Source: CAD feature listing. Evaluate the final solid. Frame: model axes, mm. A direction names the side the tool comes from. Give positions to 0.01 mm unless a question says otherwise; leave off trailing zeros. Loops run counter-clockwise (first coordinate to the right, second up) from the corner with the lowest first, then second, coordinate; pieces in that order, holes last. Notation, with made-up numbers: M 15,74 L 38,74 A35 cw 38,110 Z; hole C 42,-37 d9. An arc over 180 degrees is marked long. Put each result on its own line as item: value.
from build123d import *

# Parameters (mm, degrees)
SKETCH_3_R             = 6
EXTRUDE_1_DEPTH        = 4
FILLET_1_R             = 2
HOLE_WIZARD_M4_2_D     = 3.3
HOLE_WIZARD_M4_2_DEPTH = 11.5
HOLE_WIZARD_M4_2_TIP   = 0.991420021


with BuildPart() as part:
    # 草图3 → 凸台-拉伸1 (new body)
    with BuildSketch(Plane.XY):
        with BuildLine():
            Line((-2.5, -27), (2.5, -27))
            ThreePointArc((2.5, -27), (3.914213562, -26.414213562), (4.5, -25))
            Line((4.5, -25), (4.5, -24.5))
            ThreePointArc((4.5, -24.5), (5.085786438, -23.085786438), (6.5, -22.5))
            Line((6.5, -22.5), (10, -22.5))
            ThreePointArc((10, -22.5), (11.414213562, -21.914213562), (12, -20.5))
            Line((12, -20.5), (12, 20.5))
            ThreePointArc((12, 20.5), (11.414213562, 21.914213562), (10, 22.5))
            Line((10, 22.5), (4.5, 22.5))
            Line((4.5, 22.5), (4.5, 25))
            ThreePointArc((4.5, 25), (3.914213562, 26.414213562), (2.5, 27))
            Line((2.5, 27), (-2.5, 27))
            ThreePointArc((-2.5, 27), (-3.914213562, 26.414213562), (-4.5, 25))
            Line((-4.5, 25), (-4.5, 22.5))
            Line((-4.5, 22.5), (-10, 22.5))
            ThreePointArc((-10, 22.5), (-11.414213562, 21.914213562), (-12, 20.5))
            Line((-12, 20.5), (-12, -20.5))
            ThreePointArc((-12, -20.5), (-11.414213562, -21.914213562), (-10, -22.5))
            Line((-10, -22.5), (-6.5, -22.5))
            ThreePointArc((-6.5, -22.5), (-5.085786438, -23.085786438), (-4.5, -24.5))
            Line((-4.5, -24.5), (-4.5, -25))
            ThreePointArc((-4.5, -25), (-3.914213562, -26.414213562), (-2.5, -27))
        make_face()
        Circle(SKETCH_3_R, mode=Mode.SUBTRACT)
    extrude(amount=EXTRUDE_1_DEPTH)

    # 草图6 → M2.5 螺纹孔1 (revolve, cut)
    with BuildSketch(Plane(origin=(0, 27, 2), x_dir=(0, 0, 1), z_dir=(1, 0, 0))):
        Polygon((0, 0), (0, 7.865882135), (1.025, 7.25), (1.025, 0), align=None)
    hole_wizard_m2_5_1 = revolve(axis=Axis((0, 33.35, 2), (0, -1, 0)), mode=Mode.SUBTRACT)

    # 镜向1: M2.5 螺纹孔1 across plane
    add(hole_wizard_m2_5_1.mirror(Plane.ZX), mode=Mode.SUBTRACT)

    # 圆角1
    fillet_1_edges = [part.edges().sort_by_distance(p)[0] for p in [
        (-4.5, 22.5, 2),
        (4.5, 22.5, 2),
    ]]
    fillet(fillet_1_edges, radius=FILLET_1_R)

    # M4 螺纹孔2
    with Locations(Plane(origin=(0, 0, 0), x_dir=(-1, 0, 0), z_dir=(0, 0, -1))):
        with Locations((0, 16), (0, -16)):
            Hole(HOLE_WIZARD_M4_2_D / 2, depth=HOLE_WIZARD_M4_2_DEPTH)
            with Locations((0, 0, -(HOLE_WIZARD_M4_2_DEPTH + HOLE_WIZARD_M4_2_TIP / 2))):  # 118° drill point
                Cone(0, HOLE_WIZARD_M4_2_D / 2, HOLE_WIZARD_M4_2_TIP, mode=Mode.SUBTRACT)


solid = part.part
1. Section query B-B (y = 5.5). Output: boundary loops of the cut face in (x, z), plus the area to 3 significant figures.
Found:
outline: M -12,0 L -2.4,0 L -2.4,4 L -12,4 Z; M 2.4,0 L 12,0 L 12,4 L 2.4,4 Z
area: 76.8 mm^2
2. Access query for faces 1 (the flat face through (8, -22.5, 2)), 2 (the cylindrical face through (-0.045, 23.426, 0.976)), 3 (the flat face through (-8, -22.5, 2)). Directions: +Z, -Z, +X, -X, +Y, -Y. A direction counts if a zero-diameter tool reaches every point of the face in a straight line with its end or side. Return the directions, or none.
Found:
face 1: +Z, -Z, +X, -Y
face 2: +Y
face 3: +Z, -Z, -X, -Y
3. Section query A-A (y = 16). Output: boundary loops of the cut face in (x, z).
Found:
outline: M -12,0 L -1.65,0 L -1.65,4 L -12,4 Z; M 1.65,0 L 12,0 L 12,4 L 1.65,4 Z
4. Material intervals for line 1 (Y direction, x = 0, z = 3.1); line 2 (Y direction, x = 0, z = 1.25); line 3 (X direction, y = 24.75, z = 2) (3 decimals), sorted ascending. Write a range as from..to.
Found:
line 1: -27..-17.65, -14.35..-6, 6..14.35, 17.65..27
line 2: -19.58..-17.65, -14.35..-6, 6..14.35, 17.65..19.58
line 3: -4.5..-1.025, 1.025..4.5
5. Contact query for flat-ended pins moving along their axis: P1, Ø9.5, axis at x = 0, y = 0, coming from the +Z side; P2, Ø1, axis at x = 1.5, y = -16, coming from the +Z side; P3, Ø1, axis at x = 8, z = 2.5, coming from the -Y side; P4, Ø1.8, axis at x = -9, z = 1.5, coming from the +Y side. Output: stop coordinate, or through.
Found:
P1: through
P2: z = 4
P3: y = -22.5
P4: y = 22.5
6. Draft query along X for faces 4 (the cylindrical face through (-3.93, -26.4, 1.97)), 5 (the cylindrical face through (-0.045, -23.426, 0.976)), 6 (the cylindrical face through (3.9, -26.43, 1.97)). Return one class per face: pulls with the +X half, pulls with the -X half, needs draft (parallel to the pull), parting line crosses it, or undercut.
Found:
face 4: pulls with the -X half
face 5: undercut
face 6: pulls with the +X half
